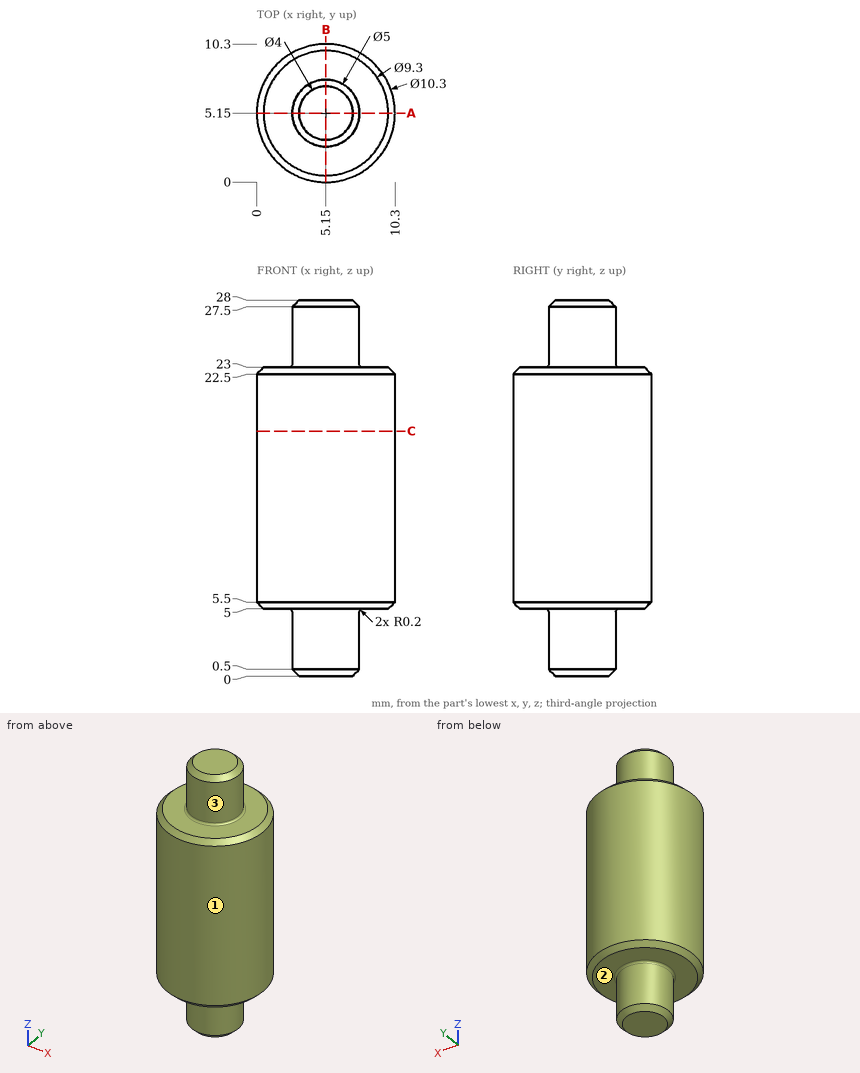
Check sheet for the drawn part. Datum: minimum x, y, z corner. Units: mm. A direction names the side the tool comes from. Round coordinates to 2 decimals unless told otherwise and drop trailing zeros. Loops run counter-clockwise (first coordinate to the right, second up) from the corner with the lowest first, then second, coordinate; pieces in that order, holes last.
Item 1: Thickness scan on line 1 (Z direction, x = 1, y = 4); line 2 (Y direction, x = 8, z = 8.75); line 3 (Y direction, x = 7.5, z = 17.25). Record the ranges inside material, lowest first.
Item 2: Cross-section at C-C on z = 18.25. Record the boundary of the cut face in (x, y), then the cut area to 3 significant figures.
Item 3: Access from +Z, -Z, +X, -X, +Y, -Y to the whole of each face (thin tool, end or side, straight path). Record for the marked faces 1, 2 and 3.
Item 4: Gauge pin test, flat ends, axial feed: pin 1 (3 mm diameter, centred on y = 1.5, z = 17, fed in from -X); pin 2 (3 mm diameter, centred on y = 2, z = 19, fed in from -X); pin 3 (1 mm diameter, centred on x = 1.5, y = 3, fed in from -Z). Record the tip position at first contact, or that the pin passes through.
Item 5: Cross-section at A-A on y = 5.15. Record the boundary of the cut face in (x, z).
Answer sheet:
1. line 1: z = 5 to 23
1. line 2: y = 0.86 to 9.44
1. line 3: y = 0.57 to 9.73
2. outline: circle Ø10.3 at (5.15, 5.15)
2. area: 83.3 mm2
3. face 1: +Z, -Z
3. face 2: -Z
3. face 3: +Z
4. pin 1: stops at x = 0.47
4. pin 2: stops at x = 0.27
4. pin 3: stops at z = 5
5. outline: (0, 5.5) - (0.5, 5) - (2.45, 5) arc R0.2 cw to (2.65, 4.8) - (2.65, 0.5) - (3.15, 0) - (7.15, 0) - (7.65, 0.5) - (7.65, 4.8) arc R0.2 cw to (7.85, 5) - (9.8, 5) - (10.3, 5.5) - (10.3, 22.5) - (9.8, 23) - (7.85, 23) arc R0.2 cw to (7.65, 23.2) - (7.65, 27.5) - (7.15, 28) - (3.15, 28) - (2.65, 27.5) - (2.65, 23.2) arc R0.2 cw to (2.45, 23) - (0.5, 23) - (0, 22.5) - close
